Here's how the part is built. I have some questions about the finished solid (model axes, mm). Face numbers are marked on the shaded views. A direction names the side the tool comes from. Coordinates: 2 decimals unless noted, no trailing zeros. Loops run counter-clockwise (first coordinate to the right, second up) from the corner with the lowest first, then second, coordinate; pieces in that order, holes last. Notation, with made-up numbers: (61.5, -33.5) -> (96.5, -33.5) arc R23 ccw to (96.5, -7.5) -> close; hole circle Ø8 at (-12.75, 77.25). An arc over 180 degrees is marked (long way). Answer as a JSON object with one key per item and string values. Group by question number.
Q1. I want a section at C-C on x = 7. Write out the boundary of the cut face in (y, z), then the cut area to 3 significant figures.
Q2. I want a section at D-D on x = -25.4. Write out the boundary of the cut face in (y, z), then the cut area to 3 significant figures.
Q3. I want a section at A-A on y = -76.2. Write out the boundary of the cut face in (x, z), then the cut area to 3 significant figures.
Q4. I need wall thicknesses on line 1 (X direction, y = -76, z = 1); line 2 (Z direction, x = -5.5, y = -77.5); line 3 (X direction, y = -65, z = 32.5). Which ranges of each line are inside material? Lowest first, please.
Q5. On a 3-axis mill with a long thin cutter (end or side, diameter ignored), from which of +Z, -Z, +X, -X, +Y, -Y can I reach the whole of each face in a straight line? I mean the marked faces 1 and 2. Say none if no direction works.
Q6. Thinking about a two-plate mould opening in X: for the marked faces 3, 4 and 5, which applies, released by +X, released by -X, zero draft, split by the parting line, or undercut?
Q7. I want a section at B-B on z = 37. Write out the boundary of the cut face in (x, y).
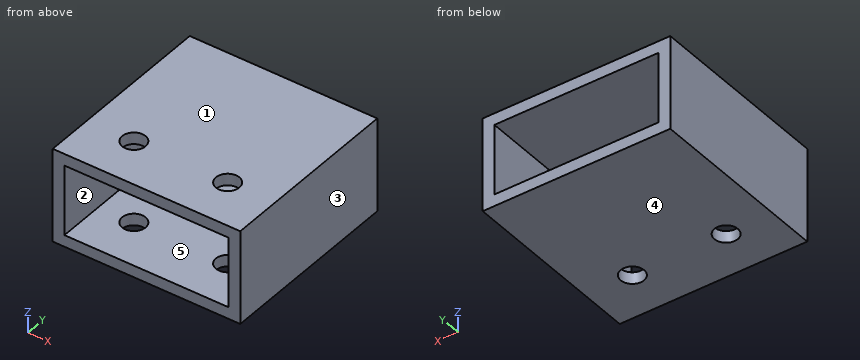
```python
from build123d import *

# Parameters (mm, degrees)
F0_W     = 101.6
F0_H     = 50.8
F0_W_2   = 88.9
F0_H_2   = 38.1
F1_DEPTH = 101.6
F2_R     = 6.35
F3_DEPTH = 50.801


with BuildPart() as f1:
    # F0 (on Front) → F1 (new body)
    with BuildSketch(Plane.XZ):
        with Locations((0, 25.4)):
            Rectangle(F0_W, F0_H)
        with Locations((0, 25.4)):
            Rectangle(F0_W_2, F0_H_2, mode=Mode.SUBTRACT)
    extrude(amount=F1_DEPTH)

    # F2 (on face) → F3 (cut, through all)
    with BuildSketch(Plane.XY.offset(50.8)):
        with Locations((25.4, -76.2)):
            Circle(F2_R)
        with Locations((-25.4, -76.2)):
            Circle(F2_R)
    extrude(amount=-F3_DEPTH, mode=Mode.SUBTRACT)


solid = f1.part
```
Result set:
{
 "1": {"outline": "(-101.6, 0) -> (0, 0) -> (0, 6.35) -> (-101.6, 6.35) -> close; (-101.6, 44.45) -> (0, 44.45) -> (0, 50.8) -> (-101.6, 50.8) -> close", "area": "1,290 mm²"},
 "2": {"outline": "(-101.6, 0) -> (-82.55, 0) -> (-82.55, 6.35) -> (-101.6, 6.35) -> close; (-101.6, 44.45) -> (-82.55, 44.45) -> (-82.55, 50.8) -> (-101.6, 50.8) -> close; (-69.85, 0) -> (0, 0) -> (0, 6.35) -> (-69.85, 6.35) -> close; (-69.85, 44.45) -> (0, 44.45) -> (0, 50.8) -> (-69.85, 50.8) -> close", "area": "1,130 mm²"},
 "3": {"outline": "(-50.8, 0) -> (-31.75, 0) -> (-31.75, 6.35) -> (-44.45, 6.35) -> (-44.45, 44.45) -> (-31.75, 44.45) -> (-31.75, 50.8) -> (-50.8, 50.8) -> close; (-19.05, 0) -> (19.05, 0) -> (19.05, 6.35) -> (-19.05, 6.35) -> close; (-19.05, 44.45) -> (19.05, 44.45) -> (19.05, 50.8) -> (-19.05, 50.8) -> close; (31.75, 0) -> (50.8, 0) -> (50.8, 50.8) -> (31.75, 50.8) -> (31.75, 44.45) -> (44.45, 44.45) -> (44.45, 6.35) -> (31.75, 6.35) -> close", "area": "1,450 mm²"},
 "4": {"line 1": "x = -50.8 to -31.75, -19.05 to 19.05, 31.75 to 50.8", "line 2": "z = 0 to 6.35, 44.45 to 50.8", "line 3": "x = -50.8 to -44.45, 44.45 to 50.8"},
 "5": {"face 1": "+Z, +X, -X, +Y, -Y", "face 2": "+Y, -Y"},
 "6": {"face 3": "released by +X", "face 4": "zero draft", "face 5": "undercut"},
 "7": {"outline": "(-50.8, -101.6) -> (-44.45, -101.6) -> (-44.45, 0) -> (-50.8, 0) -> close; (44.45, -101.6) -> (50.8, -101.6) -> (50.8, 0) -> (44.45, 0) -> close"}
}
